Design review of the part built by this model. Coordinates are the model's own, in mm. A direction names the side the tool comes from. Coordinates: 2 decimals unless noted, no trailing zeros. Write each loop counter-clockwise with the first axis right and the second up, starting at its lowest first coordinate (ties: lowest second). Pieces come first, ordered by that corner, then holes.
Q1. Take a section at B-B, the plane z = -14. State how many separate pieces and enclosed holes the cut face has, plus the area to 3 significant figures.
Q2. Take a section at D-D, the plane y = 18.5. Write out the cut boundary in (x, z).
Q3. For L1, parallel to Z at x = 9.25, y = 4.05; L2, parallel to Y at x = 0, z = 0.8; L3, parallel to Y at x = 5.5, z = -12, list the stretches that pass through material, from the lowest coordinate up.
Q4. For faces 4 (the cylindrical face through (-6.13, -15.88, -16.86)), 5 (the cylindrical face through (6.13, -5.13, -4.8)), 6 (the flat face through (-7, 6, -4)), list the 3-axis set-ups (+Z, -Z, +X, -X, +Y, -Y) from which the entire face can be reached by the end or side of a thin tool; tool diameter is ignored.
Q5. Take a section at A-A, the plane x = 9.25. Write out the cut boundary in (y, z).
Q6. For pin 1 Ø4 at (x, z) = (0, -7) entering from -Y; pin 2 Ø3.5 at (x, y) = (0, -10.5) entering from -Z; pin 3 Ø4 at (x, z) = (9, -13.5) entering from +Y, all flat-tipped, find the tip position at first contact; note any pin that passes through.
Q7. The part is to be moulded in two halves that separate along Z. For faces 1 (the flat face through (-15, 0, -16)), 2 (the cylindrical face through (-6.13, -5.13, -16.86)), 3 (the cylindrical face through (-11, -12, 1)), say which applies: released by +Z, released by -Z, zero draft, split by the parting line, or undercut.
from build123d import *

# Parameters (mm, degrees)
SKETCH_1_R           = 21.5
EXTRUDE_1_DEPTH      = 4
SKETCH_2_R           = 1.55
CUT_EXTRUDE_1_DEPTH  = 32.032845297
SKETCH_3_R           = 1.025
CUT_EXTRUDE_4_DEPTH  = 32.032845297
SKETCH_3_3_R         = 2.5
CUT_EXTRUDE_5_DEPTH  = 3
SKETCH_4_R           = 0.8
CUT_EXTRUDE_6_DEPTH  = 32.032845297
SKETCH_5_R           = 1.6
CUT_EXTRUDE_7_DEPTH  = 32.032845297
CHAMFER_1_SIZE       = 0.5
SKETCH_6_W           = 14
SKETCH_6_H           = 11.5
SKETCH_6_W_2         = 12.5
SKETCH_6_H_2         = 10
EXTRUDE_2_DEPTH      = 20
CUT_EXTRUDE_8_DEPTH  = 49.060898735
SKETCH_9_W           = 1.5
SKETCH_9_H           = 13
SKETCH_9_H_2         = 6
EXTRUDE_3_DEPTH      = 16
SKETCH_10_R          = 0.8
CUT_EXTRUDE_9_DEPTH  = 48.343316459
SKETCH_11_W          = 6
SKETCH_11_H          = 1.5
EXTRUDE_4_DEPTH      = 20
SKETCH_12_R          = 0.8
CUT_EXTRUDE_10_DEPTH = 40.50680305
RIB_12_REACH         = 38.702
SKETCH_19_WALL_W     = 86.599014246
SKETCH_19_WALL_H     = 3
RIB_14_REACH         = 38.702
SKETCH_22_WALL_W     = 86.153478968
SKETCH_22_WALL_H     = 6
RIB_44_REACH         = 43.283
SKETCH_24_WALL_W     = 100.8135827
SKETCH_24_WALL_H     = 1.5
RIB_46_REACH         = 43.283
SKETCH_25_WALL_W     = 104.02522593
SKETCH_25_WALL_H     = 1


with BuildPart() as part:
    # 草图1 → 凸台-拉伸1 (new body)
    with BuildSketch(Plane.XY):
        with Locations((-0.517890163, 0)):
            Circle(SKETCH_1_R)
    extrude(amount=EXTRUDE_1_DEPTH)

    # 草图2 → 切除-拉伸1 (cut, through all)
    with BuildSketch(Plane(origin=(0, 0, 0), x_dir=(-1, 0, 0), z_dir=(0, 0, -1))):
        Circle(SKETCH_2_R)
    extrude(amount=-CUT_EXTRUDE_1_DEPTH, mode=Mode.SUBTRACT)

    # 草图3 → 切除-拉伸4 (cut, through all)
    with BuildSketch(Plane(origin=(0, 0, 0), x_dir=(-1, 0, 0), z_dir=(0, 0, -1))):
        with Locations((12.5, 0)):
            Circle(SKETCH_3_R)
        with Locations((-12.5, 0)):
            Circle(SKETCH_3_R)
    extrude(amount=-CUT_EXTRUDE_4_DEPTH, mode=Mode.SUBTRACT)

    # 草图3<3> → 切除-拉伸5 (cut)
    with BuildSketch(Plane(origin=(0, 0, 0), x_dir=(-1, 0, 0), z_dir=(0, 0, -1))):
        with Locations((0, 10)):
            Circle(SKETCH_3_3_R)
        with Locations((12.5, -10)):
            Circle(SKETCH_3_3_R)
        with Locations(Location((-12.5, -10, 0), (0, 0, 180))):
            Circle(SKETCH_3_3_R)
    extrude(amount=-CUT_EXTRUDE_5_DEPTH, mode=Mode.SUBTRACT)

    # 草图4 → 切除-拉伸6 (cut, through all)
    with BuildSketch(Plane(origin=(0, 0, 0), x_dir=(-1, 0, 0), z_dir=(0, 0, -1))):
        with Locations((0, 10)):
            Circle(SKETCH_4_R)
        with Locations((-12.5, -10)):
            Circle(SKETCH_4_R)
        with Locations((12.5, -10)):
            Circle(SKETCH_4_R)
    extrude(amount=-CUT_EXTRUDE_6_DEPTH, mode=Mode.SUBTRACT)

    # 草图5 → 切除-拉伸7 (cut, through all)
    with BuildSketch(Plane(origin=(0, 0, 0), x_dir=(-1, 0, 0), z_dir=(0, 0, -1))):
        with Locations((0, -10.5)):
            Circle(SKETCH_5_R)
    extrude(amount=-CUT_EXTRUDE_7_DEPTH, mode=Mode.SUBTRACT)

    # 倒角1
    chamfer_1_edges = [part.edges().sort_by_distance(p)[0] for p in [
        (1.6, -10.5, 0),
    ]]
    chamfer(chamfer_1_edges, length=CHAMFER_1_SIZE)

    # 草图6 → 凸台-拉伸2 (add)
    with BuildSketch(Plane(origin=(0, 0, 0), x_dir=(-1, 0, 0), z_dir=(0, 0, -1))):
        with Locations((0, -10.5)):
            Rectangle(SKETCH_6_W, SKETCH_6_H)
        with Locations((0, -10.5)):
            Rectangle(SKETCH_6_W_2, SKETCH_6_H_2, mode=Mode.SUBTRACT)
    extrude(amount=EXTRUDE_2_DEPTH)

    # 草图8 → 切除-拉伸8 (cut, through all)
    with BuildSketch(Plane.XZ.offset(16.25)):
        with BuildLine():
            Line((-4.789423927, -3.486509961), (4.789423927, -3.486509961))
            ThreePointArc((4.789423927, -3.486509961), (6.129674245, -4.826760278), (4.789423927, -6.167010596))
            Line((4.789423927, -6.167010596), (-4.789423927, -6.167010596))
            ThreePointArc((-4.789423927, -6.167010596), (-6.129674245, -4.826760278), (-4.789423927, -3.486509961))
        make_face()
        with BuildLine():
            Line((-4.789423927, -9.486509961), (4.789423927, -9.486509961))
            ThreePointArc((4.789423927, -9.486509961), (6.129674245, -10.826760278), (4.789423927, -12.167010596))
            Line((4.789423927, -12.167010596), (-4.789423927, -12.167010596))
            ThreePointArc((-4.789423927, -12.167010596), (-6.129674245, -10.826760278), (-4.789423927, -9.486509961))
        make_face()
        with BuildLine():
            Line((-4.789423927, -15.486509961), (4.789423927, -15.486509961))
            ThreePointArc((4.789423927, -15.486509961), (6.129674245, -16.826760278), (4.789423927, -18.167010596))
            Line((4.789423927, -18.167010596), (-4.789423927, -18.167010596))
            ThreePointArc((-4.789423927, -18.167010596), (-6.129674245, -16.826760278), (-4.789423927, -15.486509961))
        make_face()
    extrude(amount=-CUT_EXTRUDE_8_DEPTH, mode=Mode.SUBTRACT)

    # 草图9 → 凸台-拉伸3 (add)
    with BuildSketch(Plane(origin=(0, 0, 0), x_dir=(-1, 0, 0), z_dir=(0, 0, -1))):
        with Locations((8.75, 3.5)):
            Rectangle(SKETCH_9_W, SKETCH_9_H)
        with Locations((15.404659184, 0.121563114)):
            Rectangle(SKETCH_9_W, SKETCH_9_H_2)
    extrude(amount=EXTRUDE_3_DEPTH)

    # 草图10 → 切除-拉伸9 (cut, through all)
    with BuildSketch(Plane.ZY.offset(16.154659184)):
        with Locations(Location((-14, 0, 0), (0, 0, 90))):
            Circle(SKETCH_10_R)
        with Locations(Location((-14, 6.5, 0), (0, 0, 90))):
            Circle(SKETCH_10_R)
    extrude(amount=-CUT_EXTRUDE_9_DEPTH, mode=Mode.SUBTRACT)

    # 草图11 → 凸台-拉伸4 (add)
    with BuildSketch(Plane(origin=(0, 0, 0), x_dir=(-1, 0, 0), z_dir=(0, 0, -1))):
        with Locations((-7.75, -3.75)):
            Rectangle(SKETCH_11_W, SKETCH_11_H)
        with Locations((-7.75, 3.75)):
            Rectangle(SKETCH_11_W, SKETCH_11_H)
    extrude(amount=EXTRUDE_4_DEPTH)

    # 草图12 → 切除-拉伸10 (cut, through all)
    with BuildSketch(Plane(origin=(0, 4.5, 0), x_dir=(1, 0, 0), z_dir=(0, 1, 0))):
        with Locations(Location((9.25, 18.5, 0), (0, 0, 90))):
            Circle(SKETCH_12_R)
        with Locations(Location((9.25, 12, 0), (0, 0, 90))):
            Circle(SKETCH_12_R)
    extrude(amount=-CUT_EXTRUDE_10_DEPTH, mode=Mode.SUBTRACT)

    # 草图19 wall → 筋12 (add, up to next)
    with BuildSketch(Plane(origin=(-17.863127863, 0, -5.330395536), x_dir=(-0.305220070795, 0, 0.952281842935), z_dir=(0.952281842935, 0, 0.305220070795)), mode=Mode.PRIVATE) as rib_12_sk1:
        Rectangle(SKETCH_19_WALL_W, SKETCH_19_WALL_H)
    rib_12_tool1 = extrude(rib_12_sk1.sketch, amount=RIB_12_REACH, mode=Mode.PRIVATE) - part.part
    add(rib_12_tool1.solids().sort_by_distance((-17.863127863, 0, -5.330395536))[0])

    # 草图22 wall → 筋14 (add, up to next)
    with BuildSketch(Plane(origin=(-6.118778075, 0, -5.034752083), x_dir=(0.350012347277, 0, 0.936745086325), z_dir=(0.936745086325, 0, -0.350012347277)), mode=Mode.PRIVATE) as rib_14_sk1:
        with Locations((0, -3)):
            Rectangle(SKETCH_22_WALL_W, SKETCH_22_WALL_H)
    rib_14_tool1 = extrude(rib_14_sk1.sketch, amount=-RIB_14_REACH, mode=Mode.PRIVATE) - part.part
    add(rib_14_tool1.solids().sort_by_distance((-6.118778075, 0, -5.034752083))[0])

    # 草图24 wall → 筋44 (add, up to next)
    with BuildSketch(Plane(origin=(7, 6.186032175, -7.946880852), x_dir=(0, 0.20754310132, 0.978225874272), z_dir=(0, -0.978225874272, 0.20754310132)), mode=Mode.PRIVATE) as rib_44_sk1:
        Rectangle(SKETCH_24_WALL_W, SKETCH_24_WALL_H)
    rib_44_tool1 = extrude(rib_44_sk1.sketch, amount=RIB_44_REACH, mode=Mode.PRIVATE) - part.part
    add(rib_44_tool1.solids().sort_by_distance((7, 6.186032175, -7.946880852))[0])

    # 草图25 wall → 筋46 (add, up to next)
    with BuildSketch(Plane(origin=(7, -6.405254219, -9.541222999), x_dir=(0, -0.195820598306, 0.980639736743), z_dir=(0, -0.980639736743, -0.195820598306)), mode=Mode.PRIVATE) as rib_46_sk1:
        with Locations((0, -0.5)):
            Rectangle(SKETCH_25_WALL_W, SKETCH_25_WALL_H)
    rib_46_tool1 = extrude(rib_46_sk1.sketch, amount=-RIB_46_REACH, mode=Mode.PRIVATE) - part.part
    add(rib_46_tool1.solids().sort_by_distance((7, -6.405254219, -9.541222999))[0])


solid = part.part
Responses:
1. separate pieces: 7
1. enclosed holes: 1
1. area: 76.9 mm2
2. outline: (-11.47, 0) - (10.44, 0) - (10.44, 4) - (-11.47, 4) - close
3. L1: z = -20 to -19.3, -17.7 to -12.8, -11.2 to 4
3. L2: y = -21.49 to -12.1, -8.9 to -1.55, 1.55 to 7.5, 12.5 to 21.49
3. L3: y = -16.25 to -15.5, -5.5 to -4.75, -4.5 to -3, 3 to 4.5
4. face 4: +Y, -Y
4. face 5: -Y
4. face 6: -Z, +Y
5. outline: (-19.15, 0) - (-4.5, 0) - (-4.5, -11.2) - (-3, -11.2) - (-3, 0) - (3, 0) - (3, -11.2) - (4.5, -11.2) - (4.5, 0) - (19.15, 0) - (19.15, 4) - (-19.15, 4) - close; (-4.5, -20) - (-3, -20) - (-3, -19.3) - (-4.5, -19.3) - close; (-4.5, -17.7) - (-3, -17.7) - (-3, -12.8) - (-4.5, -12.8) - close; (3, -20) - (4.5, -20) - (4.5, -19.3) - (3, -19.3) - close; (3, -17.7) - (4.5, -17.7) - (4.5, -12.8) - (3, -12.8) - close
6. pin 1: stops at y = -16.25
6. pin 2: stops at z = 0.35
6. pin 3: stops at y = 5.34
7. face 1: released by -Z
7. face 2: undercut
7. face 3: zero draft
